CAD build for the part. Positions are in the model's coordinates, mm. A direction names the side the tool comes from. Coordinates: 2 decimals unless noted, no trailing zeros. Loops run counter-clockwise (first coordinate to the right, second up) from the corner with the lowest first, then second, coordinate; pieces in that order, holes last. Notation, with made-up numbers: (56, -4) -> (91, -4) arc R24 cw to (91, 19) -> close; hole circle Ø1 at (-31.5, -40). An arc over 180 degrees is marked (long way). Write item = value, one per line. Start each with the question number.
(1) Pull direction X, two halves, no side cores. Call faces 1 (the face through (-60, -69.78, 1)), 2 (the face through (-115.935, -52, 1)), 3 (the face through (-43.435, -26, 1)): +X half, -X half, draft (parallel to the pull), parting line (faces both ways), or undercut.
(2) Band-saw the part on A-A (x = -14). Write the cut outline in (y, z).
(3) Tool access for faces 4 (the face through (-60, -34.78, 1)), 5 (the face through (-117, -44.78, 1)), 6 (the face through (-62.935, -74, 1)), 7 (the face through (-61.435, -71, 1)), 8 (the face through (-76.435, -79, 1)): list every direction of +Z, -Z, +X, -X, +Y, -Y with a clear straight run to the whole face (end or side of a thin tool).
(4) Band-saw the part on B-B (y = -47). Write the cut outline in (x, z), and give its area (3 significant figures).
(5) Drill centre lines: line 1 (Y direction, x = -57.5, z = 2.8); line 2 (X direction, y = -31.5, z = 1.65); line 3 (X direction, y = -32.5, z = 1.75). Where is each one in solid material? Low to high. Write a range as from..to.
(6) Flat gauge pins, fed straight in: P1, Ø1.6, axis at x = -62.5, z = 1, coming from the +Y side; P2, Ø0.8, axis at x = -58, z = 1.5, coming from the -Y side. Where does each tip first touch, or does it go through?
```python
from build123d import *

# Parameters (mm, degrees)
F1_DEPTH = 3


with BuildPart() as f1:
    # F0 (on Top) → F1 (new body)
    with BuildSketch(Plane.XY):
        Polygon((-76.435372, -27.280482), (-118.935372, -27.280482), (-118.935372, -44.780482), (-115.935372, -44.780482), (-115.935372, -59.780482), (-118.935372, -59.780482), (-118.935372, -77.280482), (-76.435372, -77.280482), (-76.435372, -80.280482), (-66.435372, -80.280482), (-66.435372, -77.280482), (-61.435372, -77.280482), (-61.435372, -75.280482), (-62.935372, -75.280482), (-62.935372, -72.780482), (-61.435372, -72.780482), (-61.435372, -69.780482), (-58.435372, -69.780482), (-58.435372, -72.780482), (-56.935372, -72.780482), (-56.935372, -75.280482), (-58.435372, -75.280482), (-58.435372, -77.280482), (-53.435372, -77.280482), (-53.435372, -80.280482), (-43.435372, -80.280482), (-43.435372, -77.280482), (-3.935372, -77.280482), (-3.935372, -27.280482), (-43.435372, -27.280482), (-43.435372, -24.280482), (-53.435372, -24.280482), (-53.435372, -27.280482), (-58.435372, -27.280482), (-58.435372, -29.280482), (-56.935372, -29.280482), (-56.935372, -31.780482), (-58.435372, -31.780482), (-58.435372, -34.780482), (-61.435372, -34.780482), (-61.435372, -31.780482), (-62.935372, -31.780482), (-62.935372, -29.280482), (-61.435372, -29.280482), (-61.435372, -27.280482), (-66.435372, -27.280482), (-66.435372, -24.280482), (-76.435372, -24.280482), align=None)
    extrude(amount=F1_DEPTH)


solid = f1.part
```
Findings below:
q1.face_1 = undercut
q1.face_2 = -X half
q1.face_3 = +X half
q2.outline = (-77.28, 0) -> (-27.28, 0) -> (-27.28, 3) -> (-77.28, 3) -> close
q3.face_4 = +Z, -Z, +Y
q3.face_5 = +Z, -Z, -X
q3.face_6 = +Z, -Z
q3.face_7 = +Z, -Z, -Y
q3.face_8 = +Z, -Z, -X, -Y
q4.outline = (-115.94, 0) -> (-3.94, 0) -> (-3.94, 3) -> (-115.94, 3) -> close
q4.area = 336 mm²
q5.line_1 = -77.28..-75.28, -72.78..-31.78, -29.28..-27.28
q5.line_2 = -118.94..-62.94, -56.94..-3.94
q5.line_3 = -118.94..-61.44, -58.44..-3.94
q6.P1 = -27.28
q6.P2 = -77.28
